Build history of the part. All positions in model axes, mm. Round coordinates to 2 decimals unless told otherwise and drop trailing zeros. Write each loop counter-clockwise with the first axis right and the second up, starting at its lowest first coordinate (ties: lowest second). Pieces come first, ordered by that corner, then holes. Notation, with made-up numbers: M -10.75,56 L 2.25,56 A16 cw 2.25,66 Z; hole C 72.25,35.25 d5. An arc over 180 degrees is marked long. Write item = value, one per line.
from build123d import *

# Parameters (mm, degrees)
SKETCH4_R           = 1
SKETCH4_R_2         = 1.5
SKETCH4_R_3         = 1.500000001
BOSS_EXTRUDE2_DEPTH = 1.5875


with BuildPart() as part:
    # Sketch4 → Boss-Extrude2 (new body)
    with BuildSketch(Plane.XY):
        with BuildLine():
            ThreePointArc((-33.472754103, -25.121469845), (-23.054804413, -30.112701264), (-11.610361031, -31.68457355))
            Line((-11.610361031, -31.68457355), (0, -32.144613372))
            Line((0, -32.144613372), (11.610361031, -31.68457355))
            ThreePointArc((11.610361031, -31.68457355), (23.054804413, -30.112701264), (33.472754103, -25.121469845))
            ThreePointArc((33.472754103, -25.121469845), (38.084735692, -20.128369992), (41.315395383, -14.148047401))
            Line((41.315395383, -14.148047401), (43.310324676, -8.545068137))
            ThreePointArc((43.310324676, -8.545068137), (44.448650445, -2.324461154), (45.212741618, 3.953110149))
            ThreePointArc((45.212741618, 3.953110149), (44.453814547, 6.519739723), (42.09374947, 7.782138432))
            ThreePointArc((42.09374947, 7.782138432), (35.962680023, 8.111048014), (29.846780415, 8.653234381))
            ThreePointArc((29.846780415, 8.653234381), (25.580679905, 10.088760175), (22.077124707, 12.914613823))
            ThreePointArc((22.077124707, 12.914613823), (19.390258386, 17.570844388), (18.500000009, 22.872464303))
            Line((18.500000009, 22.872464303), (18.500000009, 35.75))
            ThreePointArc((18.500000009, 35.75), (17.62132035, 37.87132035), (15.5, 38.750000009))
            Line((15.5, 38.750000009), (-15.5, 38.750000009))
            ThreePointArc((-15.5, 38.750000009), (-17.62132035, 37.87132035), (-18.500000009, 35.75))
            Line((-18.500000009, 35.75), (-18.500000009, 22.872464277))
            ThreePointArc((-18.500000009, 22.872464277), (-19.390258383, 17.570844381), (-22.07712469, 12.91461383))
            ThreePointArc((-22.07712469, 12.91461383), (-25.580679805, 10.088760216), (-29.846780215, 8.653234395))
            ThreePointArc((-29.846780215, 8.653234395), (-35.962679941, 8.111048017), (-42.093749505, 7.78213843))
            ThreePointArc((-42.093749505, 7.78213843), (-44.453814559, 6.519739711), (-45.212741618, 3.953110149))
            ThreePointArc((-45.212741618, 3.953110149), (-44.448650445, -2.324461154), (-43.310324676, -8.545068137))
            Line((-43.310324676, -8.545068137), (-41.315395383, -14.148047401))
            ThreePointArc((-41.315395383, -14.148047401), (-38.084735692, -20.128369992), (-33.472754103, -25.121469845))
        make_face()
        with Locations((-9.815163292, -28.866300371)):
            Circle(SKETCH4_R, mode=Mode.SUBTRACT)
        with Locations((-40.488991371, -7.557479081)):
            Circle(SKETCH4_R, mode=Mode.SUBTRACT)
        with BuildLine():
            Line((-39.916947455, -13.605513167), (-41.326325711, -9.6458687))
            ThreePointArc((-41.326325711, -9.6458687), (-38.316546684, -6.971830651), (-42.262559751, -6.172937569))
            ThreePointArc((-42.262559751, -6.172937569), (-43.119549374, -1.052504396), (-43.720300768, 4.104274139))
            ThreePointArc((-43.720300768, 4.104274139), (-43.306279922, 5.553180603), (-41.988991391, 6.284955247))
            ThreePointArc((-41.988991391, 6.284955247), (-35.815859297, 6.617706074), (-29.658025423, 7.164848598))
            ThreePointArc((-29.658025423, 7.164848598), (-26.630229039, 7.954390182), (-23.847155024, 9.384574043))
            ThreePointArc((-23.847155024, 9.384574043), (-23.125480938, 9.525676377), (-22.515405804, 9.115150267))
            ThreePointArc((-22.515405804, 9.115150267), (-20.254015304, 7.760773306), (-17.79651867, 8.714153732))
            Line((-17.79651867, 8.714153732), (-2.913646, 0.714609672))
            ThreePointArc((-2.913646, 0.714609672), (0, -3), (2.913646001, 0.714609672))
            Line((2.913646001, 0.714609672), (17.79651867, 8.714153732))
            ThreePointArc((17.79651867, 8.714153732), (20.254015126, 7.760773292), (22.515405609, 9.115149969))
            ThreePointArc((22.515405609, 9.115149969), (23.125480765, 9.52567634), (23.847155026, 9.384574041))
            ThreePointArc((23.847155026, 9.384574041), (26.630229041, 7.954390183), (29.658025423, 7.164848601))
            ThreePointArc((29.658025423, 7.164848601), (35.815859287, 6.617706075), (41.988991371, 6.284955244))
            ThreePointArc((41.988991371, 6.284955244), (43.306279914, 5.553180608), (43.720300768, 4.104274139))
            ThreePointArc((43.720300768, 4.104274139), (43.119549374, -1.052504396), (42.262559751, -6.172937569))
            ThreePointArc((42.262559751, -6.172937569), (38.316546684, -6.971830651), (41.326325712, -9.6458687))
            Line((41.326325712, -9.6458687), (39.916947456, -13.605513167))
            ThreePointArc((39.916947456, -13.605513167), (36.88563151, -19.226390572), (32.562542901, -23.926820768))
            ThreePointArc((32.562542901, -23.926820768), (22.58818115, -28.686629582), (11.638338487, -30.184834485))
            ThreePointArc((11.638338487, -30.184834485), (9.815163292, -26.616300371), (7.991988098, -30.184834485))
            ThreePointArc((7.991988098, -30.184834485), (4.00190894, -30.517536934), (0, -30.644609524))
            ThreePointArc((0, -30.644609524), (-4.00190894, -30.517536934), (-7.991988097, -30.184834485))
            ThreePointArc((-7.991988097, -30.184834485), (-9.815163292, -26.616300371), (-11.638338487, -30.184834485))
            ThreePointArc((-11.638338487, -30.184834485), (-22.58818115, -28.686629582), (-32.562542901, -23.926820768))
            ThreePointArc((-32.562542901, -23.926820768), (-36.88563151, -19.226390572), (-39.916947455, -13.605513167))
        make_face(mode=Mode.SUBTRACT)
        with Locations((9.815163292, -28.866300371)):
            Circle(SKETCH4_R, mode=Mode.SUBTRACT)
        Circle(SKETCH4_R_2, mode=Mode.SUBTRACT)
        with Locations((40.488991371, -7.557479081)):
            Circle(SKETCH4_R, mode=Mode.SUBTRACT)
        with Locations((-20.000000001, 10.750000001)):
            Circle(SKETCH4_R_3, mode=Mode.SUBTRACT)
        with Locations((-12.5, 11.133699629)):
            Circle(SKETCH4_R_2, mode=Mode.SUBTRACT)
        with BuildLine():
            ThreePointArc((-18.952977672, 14.865256843), (-17.471741936, 18.750329795), (-17.000000007, 22.881347914))
            Line((-17.000000007, 22.881347914), (-17.000000007, 31.885058019))
            ThreePointArc((-17.000000007, 31.885058019), (-16.616434483, 32.496276684), (-15.954980266, 32.784701868))
            ThreePointArc((-15.954980266, 32.784701868), (-15.728150861, 32.758688041), (-15.5, 32.749999991))
            Line((-15.5, 32.749999991), (-0.750000001, 32.749999991))
            Line((-0.750000001, 32.749999991), (-0.750000001, 2.90473751))
            ThreePointArc((-0.750000001, 2.90473751), (-1.539319977, 2.574974565), (-2.20348133, 2.035846268))
            Line((-2.20348133, 2.035846268), (-10.824171764, 6.669467376))
            ThreePointArc((-10.824171764, 6.669467376), (-11.357116861, 7.359839891), (-11.38326289, 8.231597352))
            ThreePointArc((-11.38326289, 8.231597352), (-11.323272383, 8.342575085), (-11.222961471, 8.41907763))
            ThreePointArc((-11.222961471, 8.41907763), (-10.892379956, 13.66659477), (-15.5, 11.133699629))
            ThreePointArc((-15.5, 11.133699629), (-16.184470968, 10.375365631), (-17.008738916, 10.978816797))
            ThreePointArc((-17.008738916, 10.978816797), (-17.458857736, 12.344551974), (-18.492829269, 13.343922973))
            ThreePointArc((-18.492829269, 13.343922973), (-18.498254435, 13.347040523), (-18.503662642, 13.3501874))
            ThreePointArc((-18.503662642, 13.3501874), (-19.027733875, 14.018926796), (-18.952977672, 14.865256843))
        make_face(mode=Mode.SUBTRACT)
        with Locations((-15.5, 35.75)):
            Circle(SKETCH4_R, mode=Mode.SUBTRACT)
        with BuildLine():
            Line((-12.592865853, 37.75), (-1.5, 37.75))
            Line((-1.5, 37.75), (-1.5, 33.75))
            Line((-1.5, 33.75), (-12.612506492, 33.721747011))
            ThreePointArc((-12.612506492, 33.721747011), (-11.971383706, 35.732795451), (-12.592865853, 37.75))
        make_face(mode=Mode.SUBTRACT)
        with Locations((12.5, 11.133699629)):
            Circle(SKETCH4_R_2, mode=Mode.SUBTRACT)
        with Locations((20, 10.75)):
            Circle(SKETCH4_R_2, mode=Mode.SUBTRACT)
        with BuildLine():
            Line((17.000000002, 31.88505801), (17.000000002, 22.881347906))
            ThreePointArc((17.000000002, 22.881347906), (17.471741935, 18.750329789), (18.952977675, 14.865256841))
            ThreePointArc((18.952977675, 14.865256841), (19.027733877, 14.018926793), (18.503662641, 13.350187397))
            ThreePointArc((18.503662641, 13.350187397), (18.498254436, 13.347040521), (18.492829272, 13.343922972))
            ThreePointArc((18.492829271, 13.343922974), (17.458857737, 12.344551974), (17.008738916, 10.978816797))
            ThreePointArc((17.008738916, 10.978816797), (16.184470968, 10.375365631), (15.5, 11.133699629))
            ThreePointArc((15.5, 11.133699629), (10.892379956, 13.66659477), (11.222961471, 8.41907763))
            ThreePointArc((11.222961471, 8.41907763), (11.323272383, 8.342575085), (11.38326289, 8.231597352))
            ThreePointArc((11.38326289, 8.231597352), (11.357116861, 7.359839891), (10.824171764, 6.669467376))
            Line((10.824171764, 6.669467376), (2.20348133, 2.035846268))
            ThreePointArc((2.20348133, 2.035846268), (1.539319976, 2.574974565), (0.749999999, 2.90473751))
            Line((0.749999999, 2.90473751), (0.749999999, 32.749999991))
            Line((0.749999999, 32.749999991), (15.5, 32.749999991))
            ThreePointArc((15.5, 32.749999991), (15.728150862, 32.758688041), (15.954980267, 32.784701869))
            ThreePointArc((15.954980267, 32.784701869), (16.616434482, 32.496276679), (17.000000002, 31.88505801))
        make_face(mode=Mode.SUBTRACT)
        with Locations((0, 35.75)):
            Circle(SKETCH4_R, mode=Mode.SUBTRACT)
        with BuildLine():
            Line((1.5, 33.75), (1.5, 37.75))
            Line((1.5, 37.75), (12.592865854, 37.75))
            ThreePointArc((12.592865854, 37.75), (11.971383706, 35.732795451), (12.612506492, 33.721747011))
            Line((12.612506492, 33.721747011), (1.5, 33.75))
        make_face(mode=Mode.SUBTRACT)
        with Locations((15.5, 35.75)):
            Circle(SKETCH4_R, mode=Mode.SUBTRACT)
    extrude(amount=BOSS_EXTRUDE2_DEPTH)


solid = part.part
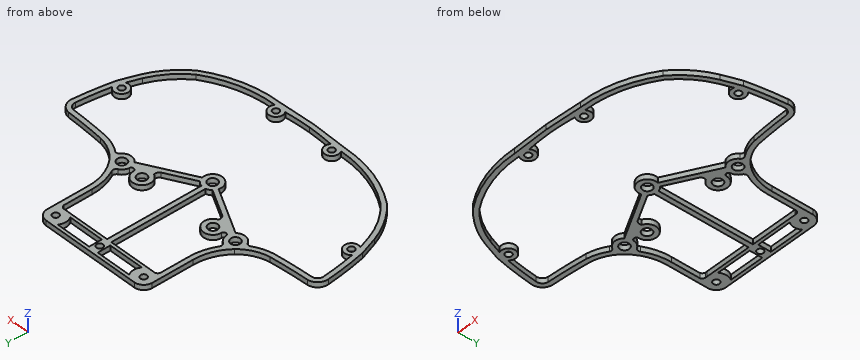
1. Band-saw the part on D-D (z = 0.25). Count the separate pieces of the cut face and the enclosed holes in it, plus the area to 3 significant figures.
Responses:
separate_pieces = 1
enclosed_holes = 17
area = 706 mm²
2. Band-saw the part on C-C (y = 16). List the corners of the cut face in (x, z).
Responses:
outline = M -20.06,0 L -18.4,0 L -18.4,1.59 L -20.06,1.59 Z; M -0.75,0 L 0.75,0 L 0.75,1.59 L -0.75,1.59 Z; M 18.4,0 L 20.06,0 L 20.06,1.59 L 18.4,1.59 Z
3. Band-saw the part on B-B (x = -27). List the corners of the cut face in (y, z), plus the area to 3 significant figures.
Responses:
outline = M -28.68,0 L -27.04,0 L -27.04,1.59 L -28.68,1.59 Z; M 7.82,0 L 9.42,0 L 9.42,1.59 L 7.82,1.59 Z
area = 5.14 mm²
4. Band-saw the part on A-A (y = 26.5). List the corners of the cut face in (x, z).
Responses:
outline = M -18.5,0 L -17,0 L -17,1.59 L -18.5,1.59 Z; M -0.75,0 L 0.75,0 L 0.75,1.59 L -0.75,1.59 Z; M 17,0 L 18.5,0 L 18.5,1.59 L 17,1.59 Z
5. Flat gauge pins, fed straight in: pin 1 (0.8 mm diameter, centred on x = 7, z = 1, fed in from -Y); pin 2 (0.5 mm diameter, centred on y = 36.5, z = 0.5, fed in from +X). Where does each tip first touch, or does it go through?
Responses:
pin_1 = -31.88
pin_2 = 18.46
6. Probe probe 1 along X at (y, z) = (25, 0.1); probe 2 along Y at (x, z) = (10.5, 1.1) (3 decimals); probe 3 along Y at (x, z) = (20, 0.65). List the from-to ranges inside material, lowest first.
Responses:
probe_1 = -18.5 to -17, -0.75 to 0.75, 17 to 18.5
probe_2 = -31.729 to -29.595, -28.138 to -26.723, 4.792 to 6.495, 8.898 to 13.37, 32.75 to 33.727, 37.75 to 38.75
probe_3 = -30.89 to -29.36, 7.75 to 9.25, 12.25 to 16.12
